Can you work these out from the model? Positions are in its coordinate system, mm. A direction names the side the tool comes from. Coordinates: 2 decimals unless noted, no trailing zeros. Write each loop counter-clockwise with the first axis right and the second up, starting at its lowest first coordinate (ties: lowest second). Pieces come first, ordered by that corner, then holes.
```python
from build123d import *

# Parameters (mm, degrees)
F3_DEPTH = 4.6736


# Not quite as in the source:
# - after a boolean that leaves OpenCascade's solid faulty, fix() repairs it


with BuildPart() as f1:
    # F0 (on Top) → F1 (revolve)
    with BuildSketch(Plane.XY):
        Polygon((-4.7498, 30.1625), (0, 30.1625), (0, 44.323), (-4.6736, 44.323), (-4.6736, 34.798), (-7.8994, 34.798), (-7.8994, 44.323), (-29.0322, 44.323), (-29.0322, 39.751), (-36.9316, 39.751), (-36.9316, 44.323), (-49.9618, 44.323), (-49.9618, 41.1734), (-62.1538, 41.1734), (-62.1538, 25.4889), (-52.6288, 25.4889), (-52.6288, 28.575), (-39.9288, 28.575), (-39.9288, 25.4889), (-30.1498, 25.4889), (-30.1498, 30.1625), (-22.225, 30.1625), (-22.225, 25.4889), (-16.8148, 25.4889), (-16.8148, 30.1625), (-11.0236, 30.1625), (-11.0236, 25.4889), (-4.7498, 25.4889), align=None)
    revolve(axis=Axis((-31.0769, 0, 0), (-1, 0, 0)))

    # F2 (on face) → F3 (cut)
    with BuildSketch(Plane.YZ):
        with BuildLine():
            ThreePointArc((-18.5166, 29.4624562527), (-9.6349948448, 33.4375190219), (0, 34.798))
            Line((0, 34.798), (0, 44.323))
            ThreePointArc((0, 44.323), (-10.9432900176, 42.950817601), (-21.209, 38.9192323665))
            Line((-21.209, 38.9192323665), (-18.5166, 29.4624562527))
        make_face()
        with BuildLine():
            Line((0, 44.323), (0, 34.798))
            ThreePointArc((0, 34.798), (9.6349948448, 33.4375190219), (18.5166, 29.4624562527))
            Line((18.5166, 29.4624562527), (21.209, 38.9192323665))
            ThreePointArc((21.209, 38.9192323665), (10.9432900176, 42.950817601), (0, 44.323))
        make_face()
    extrude(amount=-F3_DEPTH, mode=Mode.SUBTRACT)

    add(f1.part.fix(), mode=Mode.REPLACE)


solid = f1.part
```
1. If I drill on L1, parallel to Z at x = -27, y = 0; L2, parallel to X at y = 39.5, z = -17; L3, parallel to Y at x = -58, z = 0, over which ranges is the centre line in solid material (lowest first)?
2. We'd pull the mould along Z, two halves only. Please class faces 1 (the face through (-49.962, 29.3, 29.3)), 2 (the face through (-57.325, -20.227, 15.51)), 3 (the face through (-2.304, -19.882, 34.257)): released by +Z, released by -Z, zero draft, split by the parting line, or undercut.
3. Which directions (+Z, -Z, +X, -X, +Y, -Y) give clear straight access to the entire face, cutting with the end or side of a thin tool? Please do faces 4 (the face through (-2.342, -30.133, -1.326)), 5 (the face through (-56.143, -41.134, -1.81)), 6 (the face through (-26.132, -30.133, -1.326)).
4. If we section it at B-B, the plane x = -24.5: List the corners of the cut face in (y, z) for me (1 decimal).
5. If we section it at A-A, the plane y = -38.5: List the corners of the cut face in (x, z) for me.
6. I'm going to push flat-ended pins straight in: P1, Ø3, axis at y = -19.5, z = 14.5, coming from the +X side; P2, Ø3, axis at x = -16.5, y = -28.5, coming from the +Z side; P3, Ø4, axis at x = -42.5, y = -33.5, coming from the +Z side; P4, Ø1, axis at y = 31, z = 33.5, coming from the +X side. Where does each tip first touch, or does it pass through?
Answers:
1. L1: z = -44.32 to -30.16, 30.16 to 44.32
1. L2: x = -49.96 to -36.93, -29.03 to -7.9, -4.67 to 0
1. L3: y = -41.17 to -25.49, 25.49 to 41.17
2. face 1: zero draft
2. face 2: undercut
2. face 3: released by +Z
3. face 4: +X
3. face 5: -X
3. face 6: none
4. outline: circle Ø88.6 at (0, 0); hole circle Ø60.3 at (0, 0)
5. outline: (-62.15, -14.59) - (-49.96, -14.59) - (-49.96, -21.96) - (-36.93, -21.96) - (-36.93, -9.89) - (-29.03, -9.89) - (-29.03, -21.96) - (-7.9, -21.96) - (-7.9, 21.96) - (-29.03, 21.96) - (-29.03, 9.89) - (-36.93, 9.89) - (-36.93, 21.96) - (-49.96, 21.96) - (-49.96, 14.59) - (-62.15, 14.59) - close; (-4.67, -21.96) - (0, -21.96) - (0, 21.96) - (-4.67, 21.96) - close
6. P1: stops at x = -4.75
6. P2: stops at z = 35.15
6. P3: stops at z = 31.18
6. P4: passes through
